```python
from build123d import *

# Parameters (mm, degrees)
BOSS_EXTRUDE1_DEPTH      = 50.8
BOSS_EXTRUDE1_DEPTH_BACK = 31.75
SKETCH1_W                = 22.225
SKETCH1_H                = 3.175
SKETCH1_W_2              = 3.175
SKETCH1_H_2              = 47.625
SKETCH2_R                = 9.525
CUT_EXTRUDE1_DEPTH       = 3.175
SKETCH3_W                = 12.7
SKETCH3_H                = 25.4
CUT_EXTRUDE2_DEPTH       = 3.175


with BuildPart() as part:
    # Sketch1 → Boss-Extrude1 (new, two sides: drawn at the far end of the back side and taken through both)
    with BuildSketch(Plane(origin=(0, 0, 0), x_dir=(1, 0, 0), z_dir=(0, 1, 0)).offset(-BOSS_EXTRUDE1_DEPTH_BACK)):
        with Locations((1.5875, 0)):
            Rectangle(SKETCH1_W, SKETCH1_H)
        with Locations((-11.1125, 25.4)):
            Rectangle(SKETCH1_W_2, SKETCH1_H_2)
        with Locations((-11.1125, 0)):
            Rectangle(SKETCH1_W_2, SKETCH1_H)
    extrude(amount=BOSS_EXTRUDE1_DEPTH + BOSS_EXTRUDE1_DEPTH_BACK)

    # Sketch2 → Cut-Extrude1 (cut)
    with BuildSketch(Plane(origin=(-9.525, 0, 0), x_dir=(0, 0, -1), z_dir=(1, 0, 0))):
        with Locations((25.4, 19.05)):
            Circle(SKETCH2_R)
        Polygon((42.8625, 50.8), (49.2125, 44.45), (49.2125, 50.8), align=None)
        Polygon((23.8125, -31.75), (49.2125, -31.75), (49.2125, -6.35), align=None)
    extrude(amount=-CUT_EXTRUDE1_DEPTH, mode=Mode.SUBTRACT)

    # Sketch3 → Cut-Extrude2 (cut)
    with BuildSketch(Plane.XY.offset(1.5875)):
        Rectangle(SKETCH3_W, SKETCH3_H)
    extrude(amount=-CUT_EXTRUDE2_DEPTH, mode=Mode.SUBTRACT)


solid = part.part
```
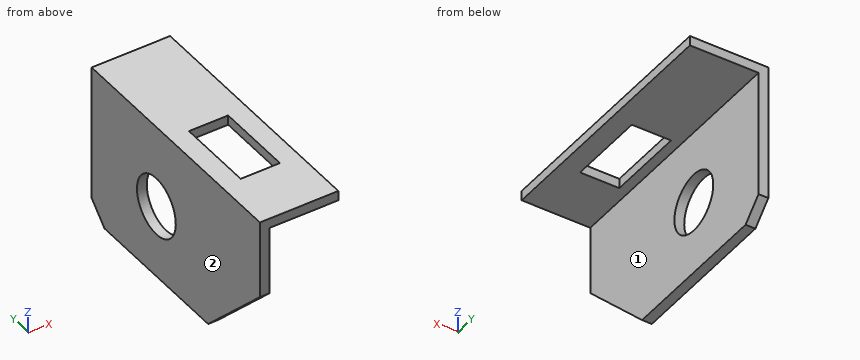
Could you check a few things on this model? Use its own coordinates, in mm. Face numbers are marked on the shaded views. A direction names the side the tool comes from. Coordinates: 2 decimals unless noted, no trailing zeros. Write each loop counter-clockwise with the first axis right and the second up, starting at its lowest first coordinate (ties: lowest second). Pieces come first, ordered by that corner, then holes. Notation, with made-up numbers: (-5, 39.5) -> (11, 39.5) arc R27 cw to (11, 67.5) -> close; hole circle Ø4 at (41.25, 21). An arc over 180 degrees is marked (long way). Write item = value, one per line. Start each with the question number.
(1) I want a section at D-D (y = 19.05). Please give me the cut outline in (x, z) (1 decimal), plus the area to 3 significant figures.
(2) I want a section at A-A (x = 2). Please give me the cut outline in (y, z), plus the area to 3 significant figures.
(3) I want a section at C-C (z = -27.5). Please give me the cut outline in (x, y) (1 decimal).
(4) I need wall thicknesses on line 1 (X direction, y = 4, z = -1); line 2 (X direction, y = 16.5, z = -6.5) (3 decimals); line 3 (Z direction, x = -3.5, y = 14). Which ranges of each line are inside material? Lowest first, please. Write a range as [from, to].
(5) Will this pin go through, and if not, where does the flat tip stop? pin 1 (24 mm diameter, centred on y = 9.5, z = -17, fed in from +X) (3 decimals).
(6) Which directions (+Z, -Z, +X, -X, +Y, -Y) give clear straight access to the entire face, cutting with the end or side of a thin tool? Please do the marked faces 1 and 2.
Result set:
q1.outline = (-12.7, -49.2) -> (-9.5, -49.2) -> (-9.5, -34.9) -> (-12.7, -34.9) -> close; (-12.7, -15.9) -> (-9.5, -15.9) -> (-9.5, -1.6) -> (12.7, -1.6) -> (12.7, 1.6) -> (-12.7, 1.6) -> close
q1.area = 171 mm2
q2.outline = (-31.75, -1.59) -> (-12.7, -1.59) -> (-12.7, 1.59) -> (-31.75, 1.59) -> close; (12.7, -1.59) -> (50.8, -1.59) -> (50.8, 1.59) -> (12.7, 1.59) -> close
q2.area = 181 mm2
q3.outline = (-12.7, -28.1) -> (-9.5, -28.1) -> (-9.5, 9.8) -> (-12.7, 9.8) -> close; (-12.7, 28.3) -> (-9.5, 28.3) -> (-9.5, 50.8) -> (-12.7, 50.8) -> close
q4.line_1 = [-12.7, -6.35], [6.35, 12.7]
q4.line_2 = [-12.7, -9.525]
q4.line_3 = [-1.59, 1.59]
q5.pin_1 = -9.525
q6.face_1 = -Z, +X, +Y, -Y
q6.face_2 = +Z, -Z, -X, +Y, -Y
